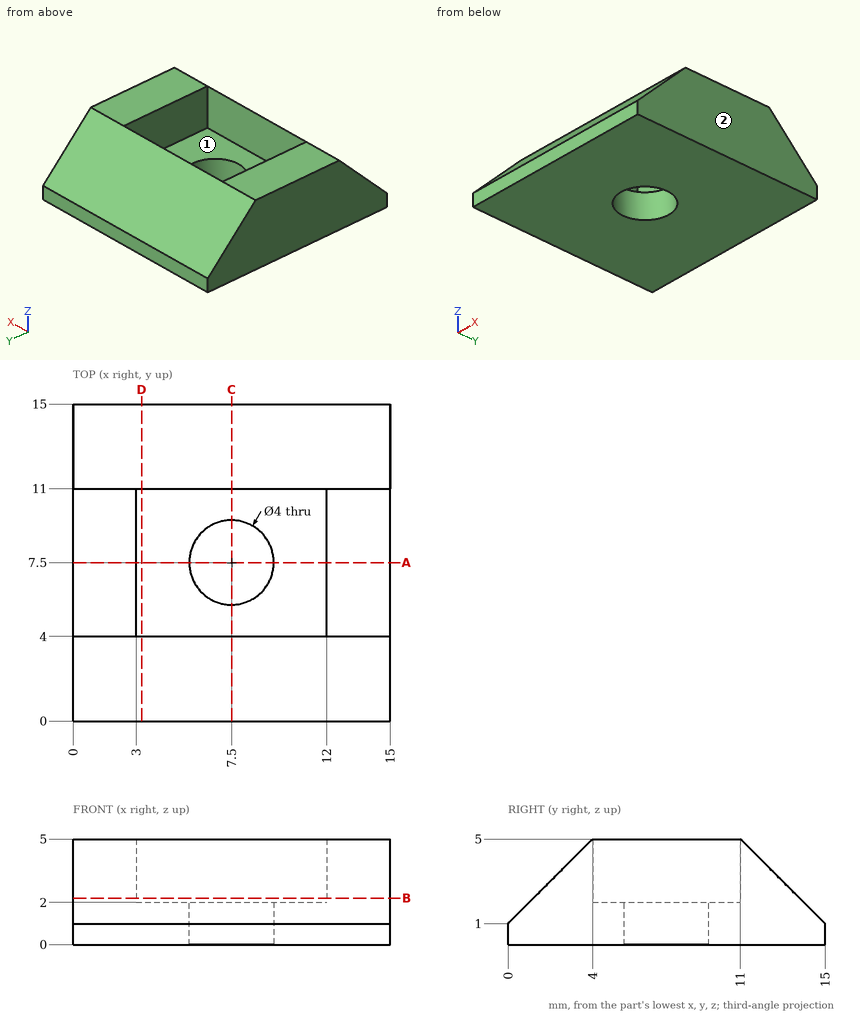
Input: dimensioned drawing with shaded views. Units: mm. Origin: part minimum x, y, z. A direction names the side the tool comes from. Round coordinates to 2 decimals unless told otherwise and drop trailing zeros. Loops run counter-clockwise (first coordinate to the right, second up) from the corner with the lowest first, then second, coordinate; pieces in that order, holes last. Notation, with made-up numbers: (83, 37) -> (116, 37) arc R25 cw to (116, 52) -> close; hole circle Ø1 at (75.25, 2). An arc over 180 degrees is marked (long way). One line per item, written item: value.
(1) Material intervals for line 1 (X direction, y = 7.5, z = 2.7); line 2 (Y direction, x = 7.5, z = 0.75); line 3 (Z direction, x = 10.5, y = 14), sorted ascending. Write a range as [from, to].
Geometry check:
line 1: [0, 3], [12, 15]
line 2: [0, 5.5], [9.5, 15]
line 3: [0, 2]
(2) Pin query (flat end, axial travel): pin 1 (2.5 mm diameter, centred on x = 7.5, y = 7.5, fed in from +Z); pin 2 (1.5 mm diameter, centred on x = 6.5, z = 4, fed in from +Y); pin 3 (4 mm diameter, centred on x = 6.5, y = 7, fed in from +Z); pin 4 (1 mm diameter, centred on x = 3.5, y = 9.5, fed in from -Z). Return the tip coordinate at first contact, or that it passes through.
Geometry check:
pin 1: through
pin 2: y = 12.75
pin 3: z = 2
pin 4: z = 0
(3) Set-up query: the marked faces 1 and 2. Return all of +Z, -Z, +X, -X, +Y, -Y with unobstructed straight access to the full face (end or side cutting, diameter ignored); none if empty.
Geometry check:
face 1: +Z
face 2: +Z, -Z, +X, +Y, -Y
(4) Section B-B (z = 2.2). Return the cut outline in (x, y), plus the area to 3 significant figures.
Geometry check:
outline: (0, 1.2) -> (15, 1.2) -> (15, 13.8) -> (0, 13.8) -> close; hole (3, 4) -> (12, 4) -> (12, 11) -> (3, 11) -> close
area: 126 mm2
(5) Section A-A (y = 7.5). Return the cut outline in (x, z).
Geometry check:
outline: (0, 0) -> (5.5, 0) -> (5.5, 2) -> (3, 2) -> (3, 5) -> (0, 5) -> close; (9.5, 0) -> (15, 0) -> (15, 5) -> (12, 5) -> (12, 2) -> (9.5, 2) -> close
(6) Section C-C (x = 7.5). Return the cut outline in (y, z).
Geometry check:
outline: (0, 0) -> (5.5, 0) -> (5.5, 2) -> (4, 2) -> (4, 5) -> (0, 1) -> close; (9.5, 0) -> (15, 0) -> (15, 1) -> (11, 5) -> (11, 2) -> (9.5, 2) -> close
(7) Section D-D (x = 3.25). Return the cut outline in (y, z), plus the area to 3 significant figures.
Geometry check:
outline: (0, 0) -> (15, 0) -> (15, 1) -> (11, 5) -> (11, 2) -> (4, 2) -> (4, 5) -> (0, 1) -> close
area: 38.0 mm2
